Read the model definition and answer for the solid it produces. Units are mm, in the model's axes. Face numbers are marked on the shaded views. A direction names the side the tool comes from. Coordinates: 2 decimals unless noted, no trailing zeros. Loops run counter-clockwise (first coordinate to the right, second up) from the corner with the lowest first, then second, coordinate; pieces in that order, holes last. Notation, with made-up numbers: (12.25, -7) -> (22.25, -7) arc R5 ccw to (22.25, -2) -> close; hole circle Ø2 at (67, -20). An arc over 180 degrees is marked (long way). Answer as a JSON object with one key per item and string values. Group by question number.
Q1. The part is cut by section A-A on y = 9. Write down the section's boundary in (x, z).
Q2. Each of these flat-tipped pins is pushed along its axis until it touches: P1, Ø4, axis at x = 8.5, z = -4, coming from the +Y side; P2, Ø1, axis at y = 7.5, z = -13.5, coming from the +X side. Where does it stop, or does it pass through?
Q3. The part is cut by section C-C on x = 10.25. Write down the section's boundary in (y, z).
Q4. The part is cut by section D-D on z = -6. Write down the section's boundary in (x, y), and give its area (3 significant figures).
Q5. The part is cut by section B-B on z = -26.25. Write down the section's boundary in (x, y), and give its area (3 significant figures).
Q6. For the marked faces 1 and 2, determine the directions among +Z, -Z, +X, -X, +Y, -Y from which every point of the face is accessible in a straight line to the end or side of a thin tool.
Q7. Straight lines are drawn through the part: line 1 along Z through (x, y) = (9, 0.85); line 2 along Z through (x, y) = (1, 9); line 3 along Y through (x, z) = (0.8, -8.75). For each, find the intervals that lie inside material, in ascending order. Write a range as [from, to].
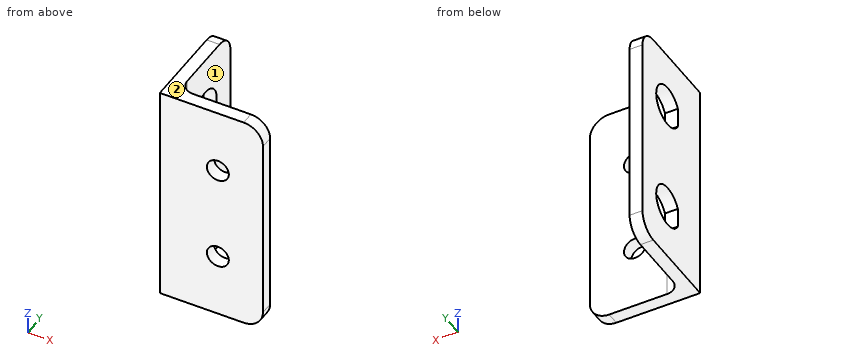
Autodesk Fusion 360 part; units mm, degrees
sketch "Sketch1" plane through (0, 0, 0) normal (0, 0, 1) x (1, 0, 0)
  line L0 (0, 0) -> (16, 0)
  line L1 (16, 0) -> (16, 2)
  line L2 (16, 2) -> (2, 2)
  line L3 (2, 2) -> (2, 16)
  line L4 (2, 16) -> (0, 16)
  line L5 (0, 16) -> (0, 0)
  dimension "d1" = 16
  dimension "d2" = 16
  dimension "d3" = 2
  dimension "d4" = 2
extrude "Extrude1" add sketch "Sketch1" against normal blind 35
sketch "Sketch2" plane through (0, 2, 0) normal (0, 1, 0) x (-1, 0, 0)
  line L0 (-2, 0) -> (-16, 0)
  line L1 (-16, 0) -> (-16, -35)
  line L2 (-16, -35) -> (-2, -35)
  line L3 (-2, -35) -> (-2, 0)
  line L4 (-9, -35) -> (-9, 0) construction
  line L5 (-16, -17.5) -> (-2, -17.5) construction
  circle A0 centre (-9, -10) radius 1.7
  circle A1 centre (-9, -25) radius 1.7
  dimension "d7" = 3.4
  dimension "d19" = 7.5
extrude "Extrude2" cut sketch "Sketch2" against normal blind 2 contours A0 | A1
sketch "Sketch3" plane through (2, 0, 0) normal (1, 0, 0) x (0, 0, -1)
  line L0 (0, 16) -> (0, 2)
  line L1 (0, 2) -> (35, 2)
  line L2 (35, 2) -> (35, 16)
  line L3 (35, 16) -> (0, 16)
  line L4 (17.5, 16) -> (17.5, 2) construction
  line L5 (0, 9) -> (35, 9) construction
  circle A0 centre (8.75, 9) radius 3.2
  line L6 (0, 12.2) -> (35, 12.2) construction
  line L7 (0, 6.2) -> (35, 6.2) construction
  line L8 (7.2008, 6.2) -> (10.2992, 6.2)
  circle A1 centre (26.25, 9) radius 3.2
  line L9 (27.7992, 6.2) -> (24.7008, 6.2)
  dimension "d10" = 6.4
  dimension "d11" = 6
  dimension "d12" = 8.75
extrude "Extrude3" cut sketch "Sketch3" against normal blind 2 contours A0 L8 | A1 L9 picked at (8.5695, 8.1846) picked at (27.2186, 9.3965)
fillet "Fillet1" radius 2 1 edges at (2, 2, -17.5)
fillet "Fillet2" radius 3 4 edges at (1, 16, -35) (1, 16, 0) (16, 1, 0) (16, 1, -35)
equation "d12 = ( 17.5 / 2 ) * 1 mm"
equation "d19 = ( 15 / 2 ) * 1 mm"
Final values:
{
 "1": {"outline": "(0, -35) -> (2, -35) -> (2, -29.45) -> (0, -29.45) -> close; (0, -23.05) -> (2, -23.05) -> (2, -11.95) -> (0, -11.95) -> close; (0, -5.55) -> (2, -5.55) -> (2, 0) -> (0, 0) -> close"},
 "2": {"P1": "stops at y = 2", "P2": "stops at x = 2"},
 "3": {"outline": "(0, -35) -> (2, -35) -> (2, -26.15) -> (0, -26.15) -> close; (0, -23.85) -> (2, -23.85) -> (2, -11.15) -> (0, -11.15) -> close; (0, -8.85) -> (2, -8.85) -> (2, 0) -> (0, 0) -> close"},
 "4": {"outline": "(0, 0) -> (16, 0) -> (16, 2) -> (4, 2) arc R2 cw to (2, 4) -> (2, 7.36) -> (0, 7.36) -> close; (0, 10.64) -> (2, 10.64) -> (2, 16) -> (0, 16) -> close", "area": "54.3 mm2"},
 "5": {"outline": "(0, 0) -> (7.85, 0) -> (7.85, 2) -> (4, 2) arc R2 cw to (2, 4) -> (2, 6.2) -> (0, 6.2) -> close; (0, 12.2) -> (2, 12.2) -> (2, 16) -> (0, 16) -> close; (10.15, 0) -> (16, 0) -> (16, 2) -> (10.15, 2) -> close", "area": "44.2 mm2"},
 "6": {"face 1": "+Z, -Z, +X, +Y", "face 2": "+Z, +X, -X, +Y, -Y"},
 "7": {"line 1": "z = [-35, -26.7], [-23.3, -11.7], [-8.3, 0]", "line 2": "z = [-35, -29.45], [-23.05, -11.95], [-5.55, 0]", "line 3": "y = [0, 6.2], [12.2, 16]"}
}
